For this review, take the finished solid that the model builds, in its own axes (mm). A direction names the side the tool comes from. Coordinates: 2 decimals unless noted, no trailing zeros. Put each result on its own line as item: value. Start each with the question number.
Item 1: The part is to be moulded in two halves that separate along X. For faces 4 (the flat face through (0, 0, 25.4)), 5 (the cylindrical face through (-0.293, -5.067, 22.269)), say which applies: +X half, -X half, draft (parallel to the pull), parting line (faces both ways), or undercut.
Item 2: For faces 1 (the flat face through (-3.3, 3.3, 0)), 2 (the flat face through (8, -2, 3.546)), 3 (the cylindrical face through (4.5, 0, 1.7)), list the 3-axis set-ups (+Z, -Z, +X, -X, +Y, -Y) from which the entire face can be reached by the end or side of a thin tool; tool diameter is ignored.
Item 3: Consider section A-A on x = 0. Give the number of separate pieces and of enclosed holes in the cut face, and give its area (3 significant figures).
Item 4: Insertion check: P1, Ø2, axis at x = -3.5, z = 14, coming from the -Y side; P2, Ø12, axis at y = 0.5, z = 13, coming from the +X side; P3, Ø8, axis at x = 7.5, z = 9, coming from the -Y side; P4, Ø6.5, axis at x = -7, y = -0.5, coming from the +Z side. Each pin has a flat end and moves straight along its axis. Give the tip position at first contact, or say it passes through.
Item 5: To check wall thickness, follow L1, parallel to Y at x = 0, z = 23; L2, parallel to Y at x = 0, z = 22; L3, parallel to Z at x = 0.75, y = 3.25. State the ranges of each line that lie inside material, in increasing order.
```python
from build123d import *

# Parameters (mm, degrees)
CUT_EXTRUDE1_DEPTH      = 0.254
CUT_EXTRUDE1_DEPTH_BACK = 29.404968727
CUT_EXTRUDE1_START      = -3.8
SKETCH5_R               = 2.999999969
SKETCH5_R_2             = 3
SKETCH6_R               = 1.75
CUT_EXTRUDE2_DEPTH      = 33.204968727
SKETCH7_R               = 2.25
SKETCH7_R_2             = 2.249999945
CUT_EXTRUDE3_DEPTH      = 33.204968727
SKETCH8_R               = 3.8
CUT_EXTRUDE4_DEPTH      = 19.05
SKETCH9_R               = 4.5
CUT_EXTRUDE5_DEPTH      = 3.5


with BuildPart() as part:
    # Loft1: read off the stored shape, not the designer's step
    # Loft1: loft between two sections, ruled curve by curve
    loft1_from = [
        Edge.make_bspline([(6.55325358, -12.371534566, 0), (7.464294458, -11.888952404, 0), (8.384566214, -11.272101526, 0), (10.134710604, -9.728764793, 0), (10.963640628, -8.800972824, 0), (12.385245025, -6.653137916, 0), (12.975801321, -5.432751611, 0), (13.784177023, -2.807609973, 0), (14, -1.404493643, 0), (14, 1.404493643, 0), (13.784177023, 2.807609973, 0), (12.975801321, 5.432751611, 0), (12.385245025, 6.653137916, 0), (10.963640628, 8.800972824, 0), (10.134710604, 9.728764793, 0), (8.384566214, 11.272101526, 0), (7.464294458, 11.888952404, 0), (6.55325358, 12.371534566, 0)], [0, 0, 0, 0, 0.125, 0.125, 0.25, 0.25, 0.375, 0.375, 0.5, 0.5, 0.625, 0.625, 0.75, 0.75, 0.875, 0.875, 1, 1, 1, 1], 3),
        Edge.make_bspline([(6.55325358, 12.371534566, 0), (5.588089256, 12.882786143, 0), (4.533369794, 13.294840206, 0), (2.318771517, 13.853790689, 0), (1.159653791, 14, 0), (-1.159653791, 14, 0), (-2.318771517, 13.853790689, 0), (-4.533369794, 13.294840206, 0), (-5.588089256, 12.882786143, 0), (-6.55325358, 12.371534566, 0)], [0, 0, 0, 0, 0.25, 0.25, 0.5, 0.5, 0.75, 0.75, 1, 1, 1, 1], 3),
        Edge.make_bspline([(-6.55325358, -12.371534566, 0), (-5.588089256, -12.882786143, 0), (-4.533369794, -13.294840206, 0), (-2.318771517, -13.853790689, 0), (-1.159653791, -14, 0), (1.159653791, -14, 0), (2.318771517, -13.853790689, 0), (4.533369794, -13.294840206, 0), (5.588089256, -12.882786143, 0), (6.55325358, -12.371534566, 0)], [0, 0, 0, 0, 0.25, 0.25, 0.5, 0.5, 0.75, 0.75, 1, 1, 1, 1], 3),
        Edge.make_bspline([(-6.55325358, 12.371534566, 0), (-7.464294458, 11.888952404, 0), (-8.384566214, 11.272101526, 0), (-10.134710604, 9.728764793, 0), (-10.963640628, 8.800972824, 0), (-12.385245025, 6.653137916, 0), (-12.975801321, 5.432751611, 0), (-13.784177023, 2.807609973, 0), (-14, 1.404493643, 0), (-14, -1.404493643, 0), (-13.784177023, -2.807609973, 0), (-12.975801321, -5.432751611, 0), (-12.385245025, -6.653137916, 0), (-10.963640628, -8.800972824, 0), (-10.134710604, -9.728764793, 0), (-8.384566214, -11.272101526, 0), (-7.464294458, -11.888952404, 0), (-6.55325358, -12.371534566, 0)], [0, 0, 0, 0, 0.125, 0.125, 0.25, 0.25, 0.375, 0.375, 0.5, 0.5, 0.625, 0.625, 0.75, 0.75, 0.875, 0.875, 1, 1, 1, 1], 3),
    ]
    loft1_to = [
        Edge.make_bspline([(6.5, -12.319, 25.4), (6.5, -11.296416667, 25.4), (6.5, -10.273833333, 25.4), (6.5, -8.228666667, 25.4), (6.5, -7.206083333, 25.4), (6.5, -5.160916667, 25.4), (6.5, -4.138333333, 25.4), (6.5, -2.093166667, 25.4), (6.5, -1.070583333, 25.4), (6.5, 0.974583333, 25.4), (6.5, 1.997166667, 25.4), (6.5, 4.042333333, 25.4), (6.5, 5.064916667, 25.4), (6.5, 7.110083333, 25.4), (6.5, 8.132666667, 25.4), (6.5, 10.177833333, 25.4), (6.5, 11.200416667, 25.4), (6.5, 12.223, 25.4)], [0, 0, 0, 0, 0.125, 0.125, 0.25, 0.25, 0.375, 0.375, 0.5, 0.5, 0.625, 0.625, 0.75, 0.75, 0.875, 0.875, 1, 1, 1, 1], 3),
        Edge.make_bspline([(6.5, 12.223, 25.4), (5.416666667, 12.223, 25.4), (4.333333333, 12.223, 25.4), (2.166666667, 12.223, 25.4), (1.083333333, 12.223, 25.4), (-1.083333333, 12.223, 25.4), (-2.166666667, 12.223, 25.4), (-4.333333333, 12.223, 25.4), (-5.416666667, 12.223, 25.4), (-6.5, 12.223, 25.4)], [0, 0, 0, 0, 0.25, 0.25, 0.5, 0.5, 0.75, 0.75, 1, 1, 1, 1], 3),
        Edge.make_bspline([(-6.5, -12.319, 25.4), (-5.416666667, -12.319, 25.4), (-4.333333333, -12.319, 25.4), (-2.166666667, -12.319, 25.4), (-1.083333333, -12.319, 25.4), (1.083333333, -12.319, 25.4), (2.166666667, -12.319, 25.4), (4.333333333, -12.319, 25.4), (5.416666667, -12.319, 25.4), (6.5, -12.319, 25.4)], [0, 0, 0, 0, 0.25, 0.25, 0.5, 0.5, 0.75, 0.75, 1, 1, 1, 1], 3),
        Edge.make_bspline([(-6.5, 12.223, 25.4), (-6.5, 11.200416667, 25.4), (-6.5, 10.177833333, 25.4), (-6.5, 8.132666667, 25.4), (-6.5, 7.110083333, 25.4), (-6.5, 5.064916667, 25.4), (-6.5, 4.042333333, 25.4), (-6.5, 1.997166667, 25.4), (-6.5, 0.974583333, 25.4), (-6.5, -1.070583333, 25.4), (-6.5, -2.093166667, 25.4), (-6.5, -4.138333333, 25.4), (-6.5, -5.160916667, 25.4), (-6.5, -7.206083333, 25.4), (-6.5, -8.228666667, 25.4), (-6.5, -10.273833333, 25.4), (-6.5, -11.296416667, 25.4), (-6.5, -12.319, 25.4)], [0, 0, 0, 0, 0.125, 0.125, 0.25, 0.25, 0.375, 0.375, 0.5, 0.5, 0.625, 0.625, 0.75, 0.75, 0.875, 0.875, 1, 1, 1, 1], 3),
    ]
    loft1 = Solid(Shell([*[Face.make_surface_from_curves(loft1_from[k], loft1_to[k]) for k in range(4)], Face(Wire(loft1_from)), Face(Wire(loft1_to))]))
    add(loft1)

    # Sketch5 → Cut-Extrude1 (cut, two sides: drawn at the far end of the back side and taken through both)
    with BuildSketch(Plane(origin=(0, 0, 0), x_dir=(-1, 0, 0), z_dir=(0, 0, -1)).offset(CUT_EXTRUDE1_START - CUT_EXTRUDE1_DEPTH_BACK)):
        with Locations(Location((-8, 0, 0), (0, 0, 300.000000342))):
            Circle(SKETCH5_R)
        with Locations(Location((8, 0, 0), (0, 0, 240))):
            Circle(SKETCH5_R_2)
    extrude(amount=CUT_EXTRUDE1_DEPTH + CUT_EXTRUDE1_DEPTH_BACK, mode=Mode.SUBTRACT)

    # Sketch6 → Cut-Extrude2 (cut, through all)
    with BuildSketch(Plane(origin=(0, 0, 0), x_dir=(-1, 0, 0), z_dir=(0, 0, -1))):
        with Locations((-8, 0)):
            Circle(SKETCH6_R)
        with Locations((8, 0)):
            Circle(SKETCH6_R)
    extrude(amount=-CUT_EXTRUDE2_DEPTH, mode=Mode.SUBTRACT)

    # Sketch7 → Cut-Extrude3 (cut, through all)
    with BuildSketch(Plane.XY.offset(25.4)):
        with Locations((0, -7.298)):
            Circle(SKETCH7_R)
        with Locations((0, 7.202)):
            Circle(SKETCH7_R_2)
    extrude(amount=-CUT_EXTRUDE3_DEPTH, mode=Mode.SUBTRACT)

    # Sketch8 → Cut-Extrude4 (cut)
    with BuildSketch(Plane(origin=(0, 0, 0), x_dir=(-1, 0, 0), z_dir=(0, 0, -1))):
        with Locations((0, -7.298)):
            Circle(SKETCH8_R)
        with Locations((0, 7.202)):
            Circle(SKETCH8_R)
    extrude(amount=-CUT_EXTRUDE4_DEPTH, mode=Mode.SUBTRACT)

    # Sketch9 → Cut-Extrude5 (cut)
    with BuildSketch(Plane(origin=(0, 0, 0), x_dir=(-1, 0, 0), z_dir=(0, 0, -1))):
        Circle(SKETCH9_R)
    extrude(amount=-CUT_EXTRUDE5_DEPTH, mode=Mode.SUBTRACT)


solid = part.part
```
Return value:
1. face 4: draft
1. face 5: undercut
2. face 1: -Z, +X, -X, +Y, -Y
2. face 2: +Z
2. face 3: -Z
3. separate pieces: 3
3. enclosed holes: 0
3. area: 296 mm^2
4. P1: y = -12.98
4. P2: x = 11.93
4. P3: y = -13.13
4. P4: z = 25.4
5. L1: -12.48 to -9.55, -5.05 to 4.95, 9.45 to 12.39
5. L2: -12.54 to -9.55, -5.05 to 4.95, 9.45 to 12.46
5. L3: 3.5 to 25.4
